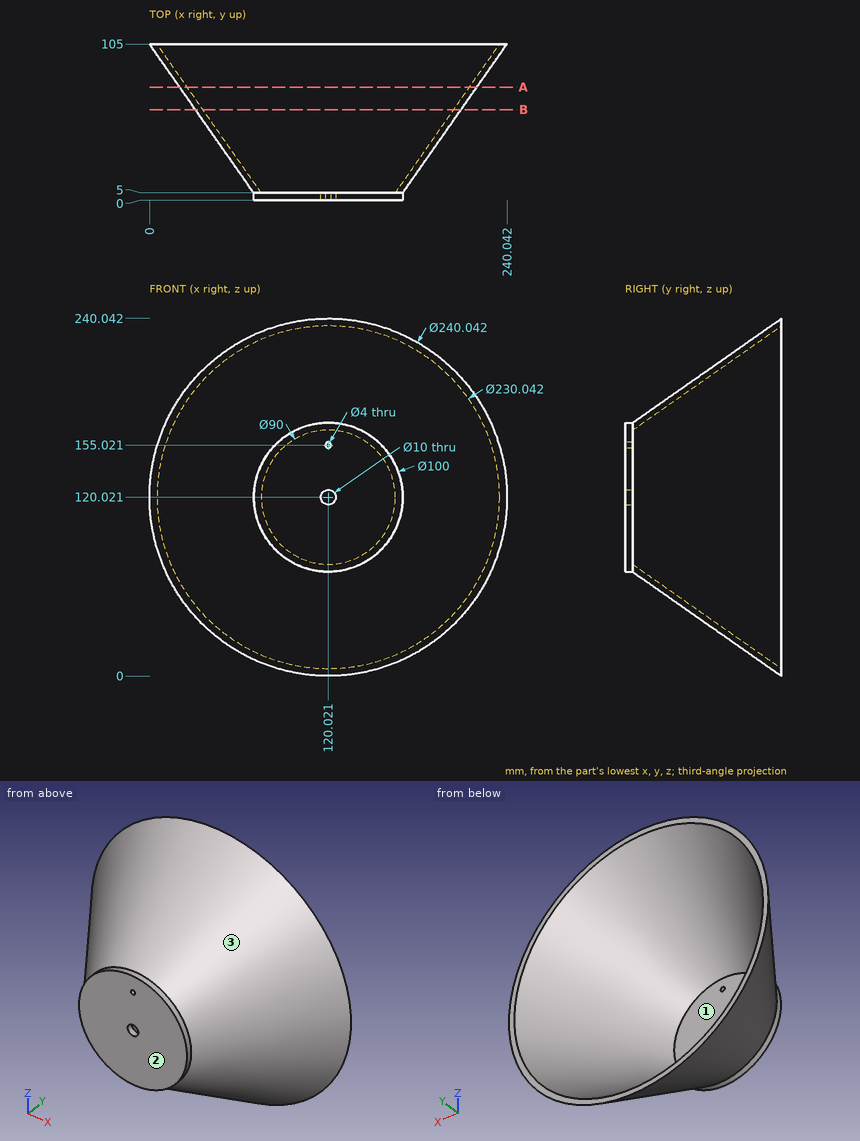
The figure shows three views and two pictorial views of one solid part (mm, origin at its lowest corner). Answer the questions. Round coordinates to 2 decimals unless told otherwise and drop trailing zeros. Loops run counter-clockwise (first coordinate to the right, second up) from the corner with the lowest first, then second, coordinate; pieces in that order, holes last. Notation, with made-up numbers: (60.5, -22.5) - (112.5, -22.5) arc R19 cw to (112.5, 14.5) - close; hole circle Ø8 at (46, 39). An arc over 180 degrees is marked (long way). Use one line per item in the form item = value. Start each with the question number.
(1) Determine the mould class of the marked faces 1, 2 and 3 for opening direction Z: +Z half, -Z half, draft (parallel to the pull), parting line (faces both ways), or undercut.
(2) Find section A-A on y = 76. Determine the outline of the cut face in (x, z) (1 decimal).
(3) Find section B-B on y = 61. Determine the outline of the cut face in (x, z).
(4) Flat-ended cylindrical pins translate along their axes: P1, Ø12, axis at x = 61, z = 71.5, coming from the +Y side; P2, Ø8, axis at x = 29.5, z = 120, coming from the -Y side (1 decimal); P3, Ø1, axis at x = 74.5, y = 14.5, coming from the -Z side (1 decimal); P4, Ø3, axis at x = 120.02, z = 155.02, coming from the +Y side. Find the tip coordinate at first contact, or state that the pin passes through.
(5) Consider line 1 (Y direction, x = 138.5, z = 146); line 2 (Z direction, x = 118, y = 71.5) (1 decimal); line 3 (X direction, y = 10, z = 123) (1 decimal). Determine where each line is inside the solid, lowest interval first.
Answer list:
q1.face_1 = undercut
q1.face_2 = draft
q1.face_3 = parting line
q2.outline = circle Ø199.4 at (120, 120); hole circle Ø189.4 at (120, 120)
q3.outline = circle Ø178.42 at (120.02, 120.02); hole circle Ø168.42 at (120.02, 120.02)
q4.P1 = 58.42
q4.P2 = 57.2
q4.P3 = 85.4
q4.P4 = through
q5.line_1 = 0 to 5
q5.line_2 = 23.5 to 28.5, 211.6 to 216.6
q5.line_3 = 66.6 to 71.6, 168.4 to 173.4
